Autodesk Inventor part; units mm, degrees
ref_plane "YZ Plane" through (0, 0, 0) normal (1, 0, 0) x (0, 1, 0)
ref_plane "XZ Plane" through (0, 0, 0) normal (0, 1, 0) x (-1, 0, 0)
ref_plane "XY Plane" through (0, 0, 0) normal (0, 0, 1) x (1, 0, 0)
sketch "Sketch1" plane through (0, 0, 0) normal (1, 0, 0) x (0, 1, 0)
  circle A0 centre (-10.828, 28.2084) radius 15.975
  circle A1 centre (108.9876, 145.8935) radius 16
  line L0 (0.3646, 16.8099) -> (120.1977, 134.4771)
  line L1 (-22.0239, 39.6037) -> (97.7741, 157.3065)
  circle A2 centre (-10.828, 28.2084) radius 20.975
  line L2 (-25.5281, 43.1703) -> (94.2699, 160.8731)
  line L3 (3.8677, 13.2422) -> (123.7008, 130.9094)
  circle A3 centre (108.9876, 145.8935) radius 21
  point P0 (0, 0)
  dimension "d0" = 5
  dimension "d1" = 5
  dimension "d2" = 5
  dimension "d3" = 5
extrude "Extrusion1" add sketch "Sketch1" along normal blind 5 contours A0 L0 A2 L1 | A2 L2 A3 L1 | L0 A3 L3 A2 | A3 L0 A1 L1 picked at (6.4932, 21.5544) picked at (91.6433, 152.5567)
fillet "Fillet1" radius 2.5 16 edges at (0, -25.792, 13.5105) (0, 63.7843, 72.0758) (0, 123.9694, 160.6089) (0, 34.3709, 102.0217) (5, -25.792, 13.5105) (5, 63.7843, 72.0758) (5, 123.9694, 160.6089) (5, 34.3709, 102.0217) (5, 120.4023, 157.1052) (5, 60.2811, 75.6435) (5, -22.2249, 17.0142) (5, 37.8751, 98.4551) (0, -22.2249, 17.0142) (0, 37.8751, 98.4551) (0, 120.4023, 157.1052) (0, 60.2811, 75.6435)
properties part number "belt"
Geometry: final body of the model. Coordinates: model frame, mm. A direction names the side the tool comes from. Round coordinates to 2 decimals unless told otherwise and drop trailing zeros. One line per item, written item: value.
(1) Pull-direction query (Y, two-part tool) for faces 4 (the cylindrical face through (4.29, 64.1, 73.44)), 5 (the cylindrical face through (4.29, 34.06, 100.66)), 6 (the cylindrical face through (4.29, 38.19, 99.82)); classes: pulls with the +Y half, pulls with the -Y half, needs draft (parallel to the pull), parting line crosses it, or undercut.
Result sheet:
face 4: pulls with the +Y half
face 5: pulls with the -Y half
face 6: undercut
(2) Line query: probe 1 along Z at (x, y) = (2.25, 109); probe 2 along Z at (x, y) = (1.25, 38.5); probe 3 along Y at (x, z) = (0.4, 146). Output: solid intervals per line, ascending. Write a range as [from, to].
Result sheet:
probe 1: [116.49, 123.46], [161.91, 166.88]
probe 2: [47.72, 53.79], [99.54, 105.61]
probe 3: [80.76, 84.63], [126.13, 128.84]
(3) Reachability of faces 1 (the cylindrical face through (0.752, 34.032, 100.689)), 2 (the cylindrical face through (4.29, 59.97, 74.28)), 3 (the cylindrical face through (0.71, 36.51, 98.17)) from +Z, -Z, +X, -X, +Y, -Y: full face, straight path, thin tool, end or side. Return the list, or none.
Result sheet:
face 1: +Z, -X, -Y
face 2: +X
face 3: -X
(4) Pin query (flat end, axial travel): P1, Ø3, axis at x = 3, z = 97.5, coming from the -Y side; P2, Ø1.5, axis at x = 4.5, y = 113.5, coming from the -Z side. Return the tip coordinate at first contact, or that it passes through.
Result sheet:
P1: y = 28.28
P2: z = 121.04
